Check sheet for the drawn part. Datum: minimum x, y, z corner. Units: mm. Round coordinates to 2 decimals unless told otherwise and drop trailing zeros. Order: outer loops, then holes, each group sorted by start corner. A loop starts at its lowest first (then second) coordinate and runs counter-clockwise, first axis right, second up. Notation, with made-up numbers: (31, 18) -> (76, 18) arc R18 ccw to (76, 40) -> close; hole circle Ø5 at (61, 72). An arc over 180 degrees is marked (long way). Answer in a Markdown table with one row per item.
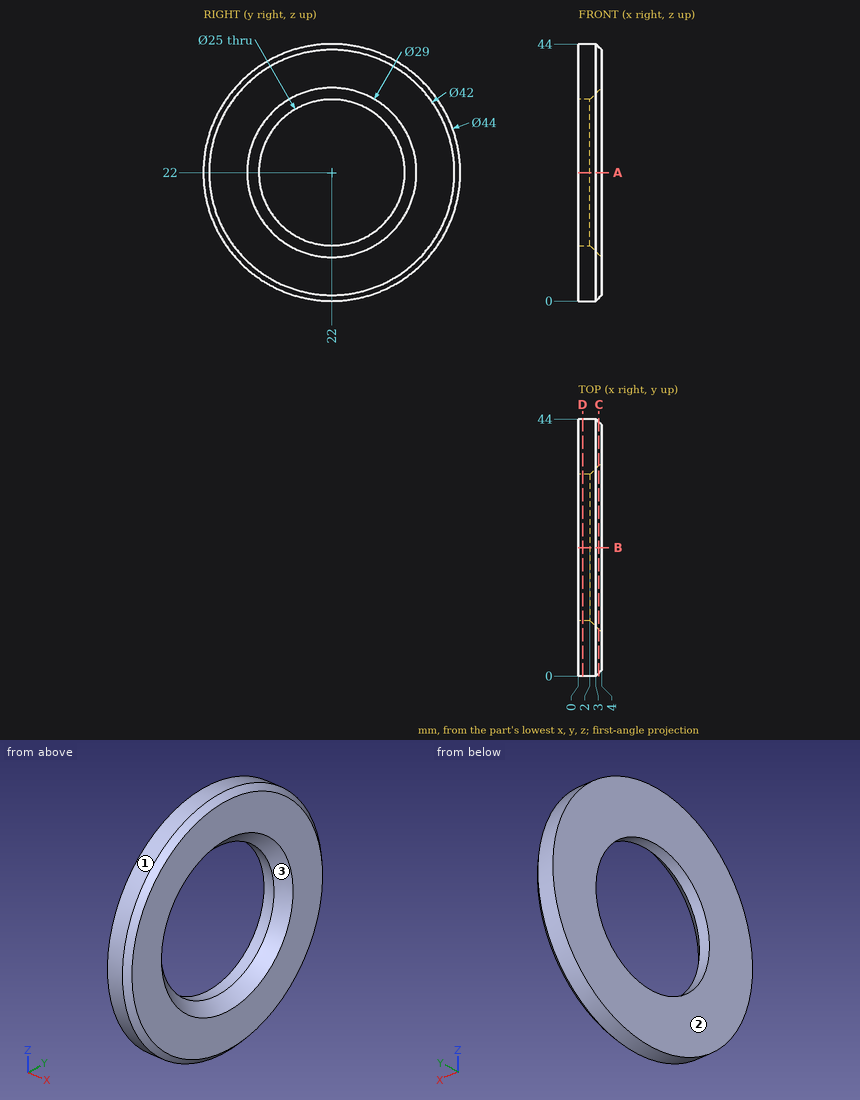
(1) Draft check along Z on the marked faces 1, 2 and 3. Enter one of: pulls with the +Z half, pulls with the -Z half, needs draft (parallel to the pull), parting line crosses it, or undercut.
Solutions:
| item | result |
|---|---|
| face 1 | parting line crosses it |
| face 2 | needs draft |
| face 3 | undercut |
(2) Depth check by flat-ended pin: pin 1 Ø3 at (y, z) = (26.5, 32.5) entering from +X; pin 2 Ø1.5 at (x, y) = (3.5, 27.5) entering from -Z. Enter the tip coordinate at first touch or a pass-through.
Solutions:
| item | result |
|---|---|
| pin 1 | x = 2.42 |
| pin 2 | z = 0.56 |
(3) Section check A-A on z = 22. Record the boundary of the cut face in (x, y), plus the area to 3 significant figures.
Solutions:
| item | result |
|---|---|
| outline | (0, 0) -> (3, 0) -> (4, 1) -> (4, 7.5) -> (2, 9.5) -> (0, 9.5) -> close; (0, 34.5) -> (2, 34.5) -> (4, 36.5) -> (4, 43) -> (3, 44) -> (0, 44) -> close |
| area | 71.0 mm^2 |
(4) Section check D-D on x = 0.75. Record the boundary of the cut face in (y, z), plus the area to 3 significant figures.
Solutions:
| item | result |
|---|---|
| outline | circle Ø44 at (22, 22); hole circle Ø25 at (22, 22) |
| area | 1,030 mm^2 |
(5) Section check C-C on x = 3.5. Record the boundary of the cut face in (y, z).
Solutions:
| item | result |
|---|---|
| outline | circle Ø43 at (22, 22); hole circle Ø28 at (22, 22) |
(6) Scan lines: probe 1 along Y at (x, z) = (0.8, 22); probe 2 along Y at (x, z) = (3.85, 25); probe 3 along Z at (x, y) = (3.55, 28). Record each from-to range of solid material in increasing order. Write a range as from..to.
Solutions:
| item | result |
|---|---|
| probe 1 | 0..9.5, 34.5..44 |
| probe 2 | 1.06..7.97, 36.03..42.94 |
| probe 3 | 1.41..9.3, 34.7..42.59 |
